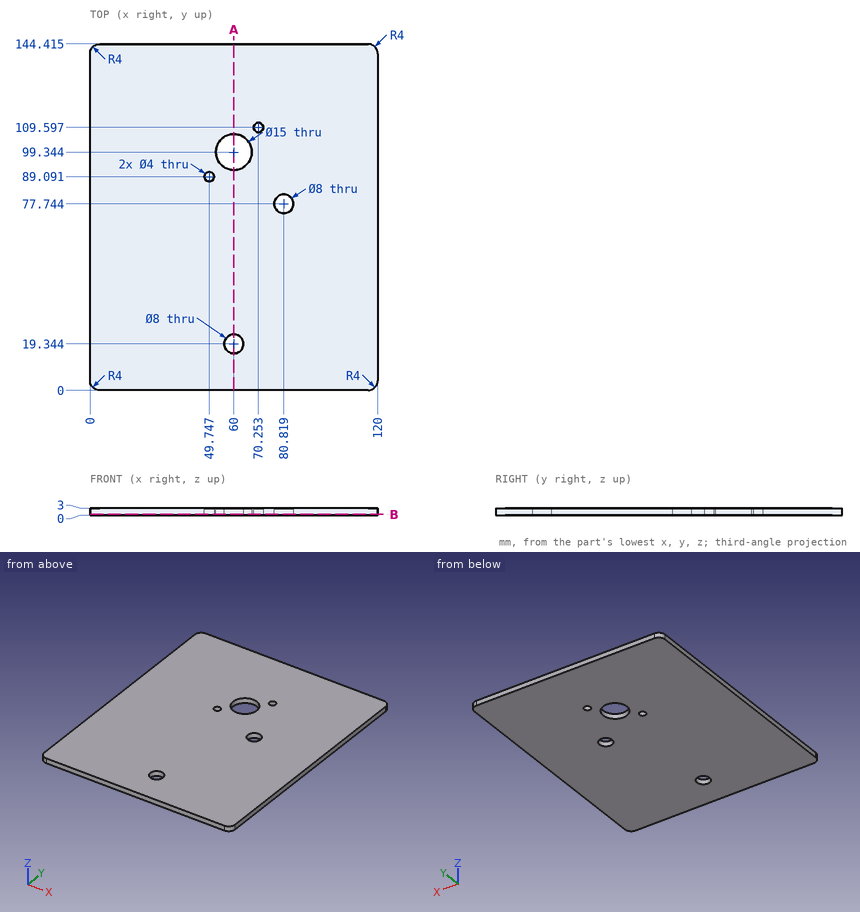
Here's the drawing with two shaded views (mm, measured from the low corner). I have some questions. Round coordinates to 2 decimals unless told otherwise and drop trailing zeros. Write each loop counter-clockwise with the first axis right and the second up, starting at its lowest first coordinate (ties: lowest second). Pieces come first, ordered by that corner, then holes. Notation, with made-up numbers: M 18.25,39.5 L 38.25,39.5 A11 ccw 38.25,46.5 Z; hole C -35.75,6 d7. An arc over 180 degrees is marked long. Answer in a Markdown table with one row per item. Add a question column.
Q1. Imagine slicing it at B-B (z = 0.5). Please give me the cut outline in (x, y) (1 decimal), then the cut area to 3 significant figures.
Q2. Will this pin go through, and if not, where does the flat tip stop? pin 1 Ø12 at (x, y) = (56, 43.5) entering from -Z.
Q3. Imagine slicing it at A-A (x = 60). Please give me the cut outline in (y, z) (1 decimal).
Q4. If I drill on line 1 (Y direction, x = 60, z = 2.4) (1 decimal); line 2 (X direction, y = 79.5, z = 1.4) (1 decimal); line 3 (Y direction, x = 58.5, z = 1.5) (1 decimal), over which ranges is the centre line in solid material (lowest first)? Write a range as from..to.
Values:
| question | item | result |
|---|---|---|
| 1 | outline | M 0,4 A4 ccw 4,0 L 116,0 A4 ccw 120,4 L 120,140.4 A4 ccw 116,144.4 L 4,144.4 A4 ccw 0,140.4 Z; hole C 49.7,89.1 d4; hole C 60,99.3 d15; hole C 60,19.3 d8; hole C 70.3,109.6 d4; hole C 80.8,77.7 d8 |
| 1 | area | 17,000 mm^2 |
| 2 | pin 1 | z = 0 |
| 3 | outline | M 0,0 L 15.3,0 L 15.3,3 L 0,3 Z; M 23.3,0 L 91.8,0 L 91.8,3 L 23.3,3 Z; M 106.8,0 L 144.4,0 L 144.4,3 L 106.8,3 Z |
| 4 | line 1 | 0..15.3, 23.3..91.8, 106.8..144.4 |
| 4 | line 2 | 0..77.2, 84.4..120 |
| 4 | line 3 | 0..15.6, 23.1..92, 106.7..144.4 |
